Could you check a few things on this model? Use its own coordinates, in mm. A direction names the side the tool comes from. Round coordinates to 2 decimals unless told otherwise and drop trailing zeros. Write each loop counter-clockwise with the first axis right and the second up, starting at its lowest first coordinate (ties: lowest second). Pieces come first, ordered by that corner, then holes. Notation, with made-up numbers: (-29.5, 78.25) -> (22.5, 78.25) arc R8 cw to (22.5, 93.25) -> close; hole circle Ø5 at (87.25, 43). An arc over 180 degrees is marked (long way). Return JSON: item names as keys, results as strings.
from build123d import *

# Parameters (mm, degrees)
EXTRUDE_THIN1_DEPTH     = 44
CUT_EXTRUDE1_REACH      = 92.628
SKETCH2_W               = 26
SKETCH2_H               = 13
CUT_EXTRUDE2_REACH      = 187.812
CUT_EXTRUDE2_END_RADIUS = 35
SKETCH3_W               = 4
SKETCH3_H               = 26


with BuildPart() as part:
    # Sketch1 → Extrude-Thin1 (new, symmetric)
    with BuildSketch(Plane.XY):
        with BuildLine():
            Line((-17.878642875, 190.536325772), (-21.038388075, 192.989081421))
            ThreePointArc((-21.038388075, 192.989081421), (-39.400871452, 200.203832377), (-58.748076809, 196.341310922))
            Line((-58.748076809, 196.341310922), (-70.262362524, 190.306310964))
            Line((-70.262362524, 190.306310964), (-70.494477907, 190.749168107))
            Line((-70.494477907, 190.749168107), (-58.980192192, 196.784168064))
            ThreePointArc((-58.980192192, 196.784168064), (-39.356598187, 200.701868398), (-20.731793619, 193.384049571))
            Line((-20.731793619, 193.384049571), (-17.572048419, 190.931293922))
            Line((-17.572048419, 190.931293922), (-17.878642875, 190.536325772))
        make_face()
    extrude(amount=EXTRUDE_THIN1_DEPTH, both=True)

    # Sketch2 → Cut-Extrude1 (cut, up to next)
    with BuildSketch(Plane(origin=(-93.623725178, 178.62640081, 0), x_dir=(0, 0, 1), z_dir=(-0.46423076597919966, 0.8857142857142849, 0)), mode=Mode.PRIVATE) as cut_extrude1_sk1:
        with Locations((0, 32.613666274)):
            Rectangle(SKETCH2_W, SKETCH2_H)
    cut_extrude1_tool1 = extrude(cut_extrude1_sk1.sketch, amount=-CUT_EXTRUDE1_REACH, mode=Mode.PRIVATE) & part.part
    add(cut_extrude1_tool1.solids().sort_by_distance((-64.737335, 193.766668, 0))[0], mode=Mode.SUBTRACT)

    # Cut-Extrude2: up to this cylinder (the profile starts outside it)
    cut_extrude2_end = Plane(origin=(-42.5, 165.341310922, 0), z_dir=(0, 0, -1)) * Cylinder(CUT_EXTRUDE2_END_RADIUS, 446.624, mode=Mode.PRIVATE)
    # Sketch3 → Cut-Extrude2 (cut, up to the surface)
    with BuildSketch(Plane(origin=(85.876233117, 110.62945285, 0), x_dir=(0.7899362999787406, -0.6131889121436371, 0), z_dir=(0.6131889121436371, 0.7899362999787406, 0)), mode=Mode.PRIVATE) as cut_extrude2_sk1:
        with Locations((-132.957751326, 0)):
            Rectangle(SKETCH3_W, SKETCH3_H)
    cut_extrude2_tool1 = extrude(cut_extrude2_sk1.sketch, amount=-CUT_EXTRUDE2_REACH, mode=Mode.PRIVATE) - cut_extrude2_end
    add(cut_extrude2_tool1.solids().sort_by_distance((-19.151921, 192.157672, 0))[0], mode=Mode.SUBTRACT)


solid = part.part
1) I want a section at B-B, the plane z = -31. Please give me the cut outline in (x, y).
Return value:
{"outline": "(-70.49, 190.75) -> (-70.26, 190.31) -> (-58.75, 196.34) arc R35 cw to (-21.04, 192.99) -> (-17.88, 190.54) -> (-17.57, 190.93) -> (-20.73, 193.38) arc R35.5 ccw to (-58.98, 196.78) -> close"}
2) For faces 1 (the face through (-39.64, 200.726, 0.616)), 2 (the face through (-19.44, 191.75, -28.28)), which set-ups out of +Z, -Z, +X, -X, +Y, -Y let a thin tool reach every point of the face, with its end or its side?
Return value:
{"face 1": "+Z, -Z, +Y", "face 2": "+Z, -Z, -Y"}
3) Thinking about a two-plate mould opening in X: for faces 3 (the face through (-64.42, 193.37, -28.28)), 4 (the face through (-19.3, 192, -13)), 5 (the face through (-19.17, 192.17, 28.72)), 6 (the face through (-39.122, 200.178, 0.616)), which applies, pulls with the +X half, pulls with the -X half, needs draft (parallel to the pull), parting line crosses it, or undercut?
Return value:
{"face 3": "undercut", "face 4": "needs draft", "face 5": "pulls with the +X half", "face 6": "undercut"}
4) I want a section at A-A, the plane y = 198. Please give me the cut outline in (x, z).
Return value:
{"outline": "(-56.42, -44) -> (-55.09, -44) -> (-55.09, 44) -> (-56.42, 44) -> close; (-29.91, -44) -> (-28.58, -44) -> (-28.58, 44) -> (-29.91, 44) -> close"}
5) If I drill on probe 1 along X at (y, z) = (193.25, -38.5); probe 2 along X at (y, z) = (195, -16); probe 3 along Y at (x, z) = (-50, 14), over which ranges is the centre line in solid material (lowest first)? Write a range as [from, to].
Return value:
{"probe 1": "[-65.72, -64.65], [-21.38, -20.56]", "probe 2": "[-62.38, -61.31], [-23.92, -22.99]", "probe 3": "[199.53, 200.04]"}
6) I want a section at D-D, the plane z = 11. Please give me the cut outline in (x, y).
Return value:
{"outline": "(-58.98, 196.78) -> (-58.75, 196.34) arc R35 cw to (-21.04, 192.99) -> (-20.73, 193.38) arc R35.5 ccw to start"}
7) I want a section at C-C, the plane x = -61. Please give me the cut outline in (y, z), and give its area (3 significant figures).
Return value:
{"outline": "(195.16, -44) -> (195.73, -44) -> (195.73, -13) -> (195.16, -13) -> close; (195.16, 13) -> (195.73, 13) -> (195.73, 44) -> (195.16, 44) -> close", "area": "35.0 mm²"}
8) Will these pins go through, and if not, where does the flat tip stop? pin 1 Ø5 at (x, z) = (-51, 28.5) entering from +Y; pin 2 Ø2 at (x, y) = (-59, 199.5) entering from +Z; pin 3 Ø10 at (x, z) = (-32, -26) entering from +Y; pin 4 Ø5 at (y, z) = (196, 29) entering from +X.
Return value:
{"pin 1": "y = 200.33", "pin 2": "through", "pin 3": "y = 200.41", "pin 4": "x = -20.88"}
